```python
from build123d import *

# Parameters (mm, degrees)
SKETCH1_R                = 250
SKETCH1_R_2              = 170
BOSS_EXTRUDE1_DEPTH      = 200
BOSS_EXTRUDE1_DEPTH_BACK = 50
SKETCH2_R                = 250
BOSS_EXTRUDE3_DEPTH      = 50
BOSS_EXTRUDE4_START      = -350
BOSS_EXTRUDE4_DEPTH      = 700


with BuildPart() as part:
    # Sketch1 → Boss-Extrude1 (new body, two sides)
    with BuildSketch(Plane.XY) as boss_extrude1_sk:
        Circle(SKETCH1_R)
        Circle(SKETCH1_R_2, mode=Mode.SUBTRACT)
    extrude(amount=BOSS_EXTRUDE1_DEPTH)
    extrude(boss_extrude1_sk.sketch, amount=-BOSS_EXTRUDE1_DEPTH_BACK)

    # Sketch2 → Boss-Extrude3 (add)
    with BuildSketch(Plane.XY):
        with BuildLine():
            Line((-650, 770), (-650, 321.130814467))
            ThreePointArc((-650, 321.130814467), (0, -725), (650, 321.130814467))
            Line((650, 321.130814467), (650, 770))
            Line((650, 770), (-650, 770))
        make_face()
        Circle(SKETCH2_R, mode=Mode.SUBTRACT)
    extrude(amount=-BOSS_EXTRUDE3_DEPTH)


with BuildPart() as body_2:
    # Mirror9: mirrored copy
    add(part.part.mirror(Plane.XY.offset(-400)))


with BuildPart() as part_1:
    add(part.part)

    add(body_2.part)  # Boss-Extrude4 merges body 2
    # Sketch4 → Boss-Extrude4 (add)
    with BuildSketch(Plane.XY.offset(-400).offset(BOSS_EXTRUDE4_START)):
        with BuildLine():
            Line((-600, 770), (-600, 309.232921921))
            ThreePointArc((-600, 309.232921921), (0, -675), (600, 309.232921921))
            Line((600, 309.232921921), (600, 770))
            Line((600, 770), (650, 770))
            Line((650, 770), (650, 321.130814467))
            ThreePointArc((650, 321.130814467), (0, -725), (-650, 321.130814467))
            Line((-650, 321.130814467), (-650, 770))
            Line((-650, 770), (-600, 770))
        make_face()
    extrude(amount=BOSS_EXTRUDE4_DEPTH)


solid = part_1.part
```
Geometry: final body of the model. Coordinates: model frame, mm. A direction names the side the tool comes from. Give positions to 0.01 mm unless a question says otherwise; leave off trailing zeros. Loops run counter-clockwise (first coordinate to the right, second up) from the corner with the lowest first, then second, coordinate; pieces in that order, holes last. Notation, with made-up numbers: (0, 72.5) -> (44, 72.5) arc R20 cw to (44, 99.5) -> close; hole circle Ø10 at (34, -5). An arc over 180 degrees is marked (long way). Return JSON: item names as keys, results as strings.
Item 1: Access query for faces 4 (the cylindrical face through (-249.76, 10.99, 101.4)), 5 (the flat face through (600, 536, -405)), 6 (the cylindrical face through (-19.338, -674.723, -404.9)). Directions: +Z, -Z, +X, -X, +Y, -Y. A direction counts if a zero-diameter tool reaches every point of the face in a straight line with its end or side. Return the directions, or none.
Filled in:
{"face 4": "+Z", "face 5": "+Y", "face 6": "none"}
Item 2: Section B-B, the plane y = 542. Output: boundary loops of the cut face in (x, z).
Filled in:
{"outline": "(-650, -800) -> (650, -800) -> (650, 0) -> (-650, 0) -> close; hole (-600, -750) -> (600, -750) -> (600, -50) -> (-600, -50) -> close"}
Item 3: Section C-C, the plane y = 0. Output: boundary loops of the cut face in (x, z).
Filled in:
{"outline": "(-725, -800) -> (-250, -800) -> (-250, -1000) -> (-170, -1000) -> (-170, -750) -> (-675, -750) -> (-675, -50) -> (-170, -50) -> (-170, 200) -> (-250, 200) -> (-250, 0) -> (-725, 0) -> close; (170, -1000) -> (250, -1000) -> (250, -800) -> (725, -800) -> (725, 0) -> (250, 0) -> (250, 200) -> (170, 200) -> (170, -50) -> (675, -50) -> (675, -750) -> (170, -750) -> close"}
Item 4: Line query: line 1 (Y direction, x = 0, z = -14); line 2 (Z direction, x = -106, y = 649); line 3 (X direction, y = 0, z = -525). Output: solid intervals per line, ascending.
Filled in:
{"line 1": "-725 to -170, 170 to 770", "line 2": "-800 to -750, -50 to 0", "line 3": "-725 to -675, 675 to 725"}
Item 5: Pin query (flat end, axial travel): P1, Ø15, axis at y = 514, z = -37.5, coming from the +X side; P2, Ø1, axis at x = -424.5, z = -553.5, coming from the +Y side; P3, Ø1.5, axis at x = 38.5, y = 586.5, coming from the +Z side. Return the tip coordinate at first contact, or that it passes through.
Filled in:
{"P1": "x = 650", "P2": "y = -524.4", "P3": "z = 0"}
Item 6: Mould query, pull axis Z, two halves, no side actions, for faces 1 (the flat face through (-600, 543, -405)), 2 (the cylindrical face through (-134.91, -103.44, -876.75)), 3 (the flat face through (-171, 199, 0)). Classes: released by +Z, released by -Z, zero draft, split by the parting line, or undercut.
Filled in:
{"face 1": "undercut", "face 2": "zero draft", "face 3": "released by +Z"}
Item 7: Section D-D, the plane z = -459.5. Output: boundary loops of the cut face in (x, y), plus the area to 3 significant figures.
Filled in:
{"outline": "(-650, 321.13) arc R725 ccw (long way) to (650, 321.13) -> (650, 770) -> (600, 770) -> (600, 309.23) arc R675 cw (long way) to (-600, 309.23) -> (-600, 770) -> (-650, 770) -> close", "area": "188,000 mm^2"}
Item 8: Section A-A, the plane x = 0. Output: boundary loops of the cut face in (y, z), plus the area to 4 significant figures.
Filled in:
{"outline": "(-725, -800) -> (-250, -800) -> (-250, -1000) -> (-170, -1000) -> (-170, -750) -> (-675, -750) -> (-675, -50) -> (-170, -50) -> (-170, 200) -> (-250, 200) -> (-250, 0) -> (-725, 0) -> close; (170, -1000) -> (250, -1000) -> (250, -800) -> (770, -800) -> (770, -750) -> (170, -750) -> close; (170, -50) -> (770, -50) -> (770, 0) -> (250, 0) -> (250, 200) -> (170, 200) -> close", "area": "214,500 mm^2"}
